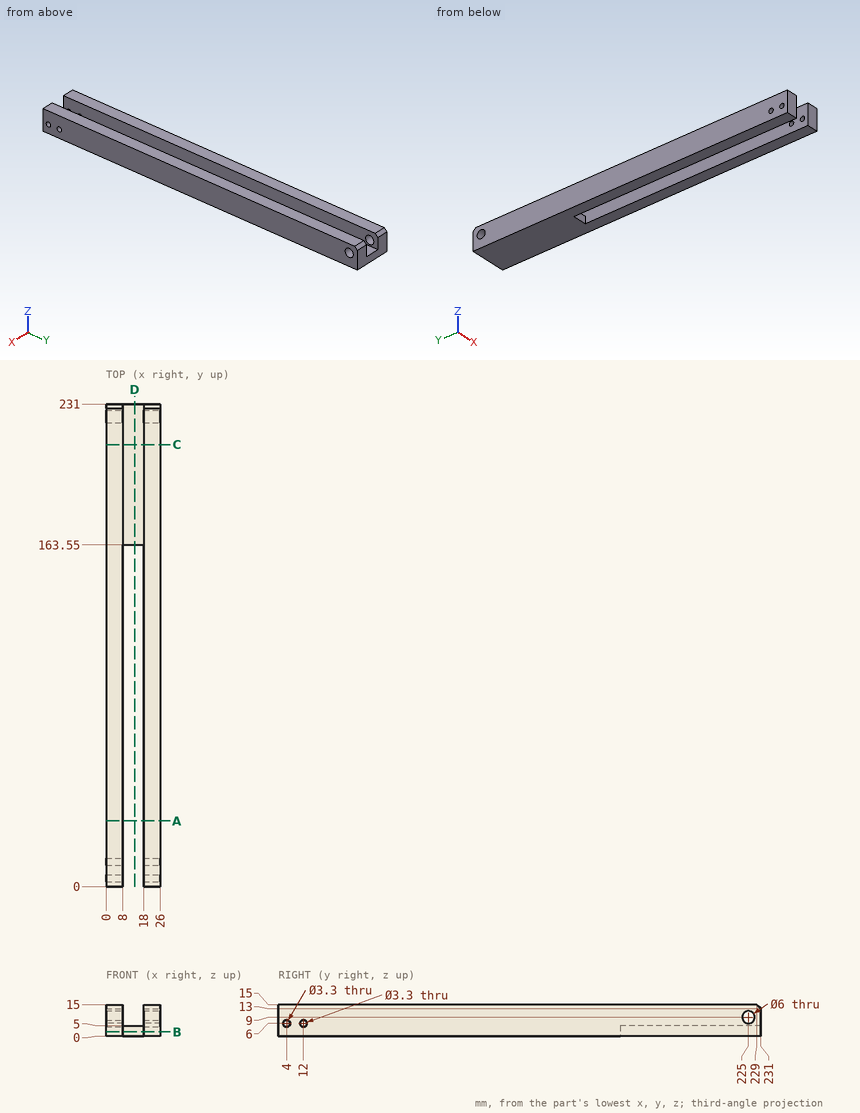
Study the drawing (mm; zero at the part's minimum x, y, z) and answer. Round coordinates to 2 decimals unless told otherwise and drop trailing zeros. Loops run counter-clockwise (first coordinate to the right, second up) from the corner with the lowest first, then second, coordinate; pieces in that order, holes last.
Q1. Section D-D, the plane x = 13.75 is taken. Determine the outline of the cut face in (y, z).
Q2. Section B-B, the plane z = 2 is taken. Determine the outline of the cut face in (x, y), then the cut area to 3 significant figures.
Q3. Section C-C, the plane y = 211.5 is taken. Determine the outline of the cut face in (x, z).
Q4. Section A-A, the plane y = 31.5 is taken. Determine the outline of the cut face in (x, z).
Q5. Find the intervals of material crossed by line 1 (Y direction, x = 21, z = 9); line 2 (X direction, y = 211, z = 7.5); line 3 (Y direction, x = 2.5, z = 6.75), in increasing order.
Q6. Given pin 1 Ø2 at (x, z) = (14, 4.5) entering from -Y; pin 2 Ø3 at (y, z) = (12, 6) entering from -X; pin 3 Ø3 at (x, y) = (11, 182.5) entering from +Z, each flat-ended and moving along its own axis, determine where each tip first touches the part or whether it passes through.
Completed:
1. outline: (163.55, 0) - (231, 0) - (231, 5) - (163.55, 5) - close
2. outline: (0, 0) - (8, 0) - (8, 163.55) - (18, 163.55) - (18, 0) - (26, 0) - (26, 231) - (0, 231) - close
2. area: 4,370 mm2
3. outline: (0, 0) - (26, 0) - (26, 15) - (18, 15) - (18, 5) - (8, 5) - (8, 15) - (0, 15) - close
4. outline: (0, 0) - (8, 0) - (8, 15) - (0, 15) - close; (18, 0) - (26, 0) - (26, 15) - (18, 15) - close
5. line 1: y = 0 to 222, 228 to 231
5. line 2: x = 0 to 8, 18 to 26
5. line 3: y = 0 to 2.53, 5.47 to 10.53, 13.47 to 223.02, 226.98 to 231
6. pin 1: stops at y = 163.55
6. pin 2: passes through
6. pin 3: stops at z = 5
